Design review of the part built by this model. Coordinates are the model's own, in mm. Face numbers are marked on the shaded views. A direction names the side the tool comes from. Give positions to 0.01 mm unless a question says otherwise; leave off trailing zeros. Loops run counter-clockwise (first coordinate to the right, second up) from the corner with the lowest first, then second, coordinate; pieces in that order, holes last. Notation, with made-up numbers: (50.5, 63.25) - (62.5, 63.25) arc R13 ccw to (62.5, 81.25) - close; hole circle Ø11 at (-13, 41.25). An arc over 180 degrees is marked (long way). Write each question's results on one line, items separated by ' | '.
from build123d import *

# Parameters (mm, degrees)
F2_R     = 4
F3_R     = 1
F4_R     = 2
F5_DEPTH = 25


with BuildPart() as f1:
    # F0 (on Top) → F1 (revolve)
    with BuildSketch(Plane.XY):
        with BuildLine():
            Line((37.5, -2.6), (37.5, 0))
            Line((37.5, 0), (46.8, 0))
            Line((46.8, 0), (46.8, 0.65))
            Line((46.8, 0.65), (38.4, 0.65))
            Line((38.4, 0.65), (38.4, 2.3))
            Line((38.4, 2.3), (34.8, 2.3))
            Line((34.8, 2.3), (34.8, 7))
            Line((34.8, 7), (21.576792, 14.108865))
            Line((21.576792, 14.108865), (18.7, 17))
            Line((18.7, 17), (18.7, 33))
            Line((18.7, 33), (0, 33))
            Line((0, 33), (0, 7.885643))
            ThreePointArc((0, 7.885643), (5.193057, 8.584234), (10.016886, 10.630338))
            Line((10.016886, 10.630338), (32.484462, 0))
            Line((32.484462, 0), (35.5, 0))
            Line((35.5, 0), (35.5, -2.6))
            Line((35.5, -2.6), (37.5, -2.6))
        make_face()
    revolve(axis=Axis((0, 27.784977, 0), (0, 1, 0)))

    # F2
    f2_edges = [f1.edges().sort_by_distance(p)[0] for p in [
        (-18.7, 33, 0),
    ]]
    fillet(f2_edges, radius=F2_R)

    # F3
    f3_edges = [f1.edges().sort_by_distance(p)[0] for p in [
        (-34.8, 7, 0),
        (-34.8, 2.3, 0),
    ]]
    fillet(f3_edges, radius=F3_R)

    # F4 (on face) → F5 (cut)
    with BuildSketch(Plane.XZ):
        with BuildLine():
            ThreePointArc((0, -46.8), (33.092597, -33.092597), (46.8, 0))
            ThreePointArc((46.8, 0), (46.300332, -3.839319), (44.834617, -7.422853))
            ThreePointArc((44.834617, -7.422853), (28.647845, -28.647845), (7.422853, -44.834618))
            ThreePointArc((7.422853, -44.834618), (3.839319, -46.300332), (0, -46.8))
        make_face()
        with BuildLine():
            ThreePointArc((-44.834618, -7.422853), (-46.300332, -3.839319), (-46.8, 0))
            ThreePointArc((-46.8, 0), (-33.092597, -33.092597), (0, -46.8))
            ThreePointArc((0, -46.8), (-3.839319, -46.300332), (-7.422853, -44.834618))
            ThreePointArc((-7.422853, -44.834618), (-28.647845, -28.647845), (-44.834618, -7.422853))
        make_face()
        with BuildLine():
            ThreePointArc((-7.422852, 44.834618), (-3.839319, 46.300332), (0, 46.8))
            ThreePointArc((0, 46.8), (-33.092597, 33.092597), (-46.8, 0))
            ThreePointArc((-46.8, 0), (-46.300332, 3.839319), (-44.834618, 7.422853))
            ThreePointArc((-44.834618, 7.422853), (-28.647845, 28.647845), (-7.422852, 44.834618))
        make_face()
        with BuildLine():
            ThreePointArc((0, 46.8), (3.839319, 46.300332), (7.422853, 44.834618))
            ThreePointArc((7.422853, 44.834618), (28.647845, 28.647845), (44.834618, 7.422853))
            ThreePointArc((44.834618, 7.422853), (46.300332, 3.839319), (46.8, 0))
            ThreePointArc((46.8, 0), (33.092597, 33.092597), (0, 46.8))
        make_face()
        with Locations((0, -42)):
            Circle(F4_R)
        with Locations((0, 42)):
            Circle(F4_R)
        with Locations((-42, 0)):
            Circle(F4_R)
        with Locations((42, 0)):
            Circle(F4_R)
    extrude(amount=-F5_DEPTH, mode=Mode.SUBTRACT)


solid = f1.part
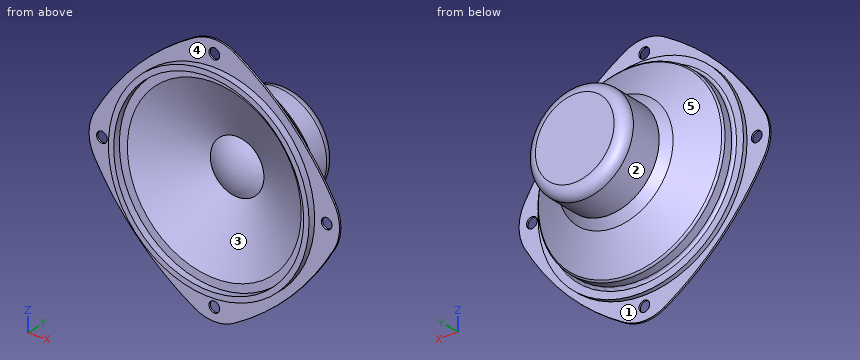
(1) Take a section at A-A on x = -42. Give the boundary of the cut face in (y, z).
Answers below:
outline: (0, -12.1) - (0.65, -12.1) - (0.65, -2) - (0, -2) - close; (0, 2) - (0.65, 2) - (0.65, 12.1) - (0, 12.1) - close
(2) Wall thickness on line 1 along Z through (x, y) = (0, -1.6); line 2 along Z through (x, y) = (-3, 1); line 3 along Z through (x, y) = (15, 29.5): over which ranges is each line inside the solid? List them lowest first. Write a range as from..to.
Answers below:
line 1: -37.5..-35.5, 35.5..37.5 | line 2: -38.28..-30.22, 30.22..38.28 | line 3: -11.11..11.11
(3) Insertion check: P1, Ø6.5, axis at x = 0, z = -42, coming from the +Y side; P2, Ø12, axis at y = 1, z = -36.5, coming from the +X side; P3, Ø12, axis at x = -14.5, y = 24, coming from the +Z side; P4, Ø3, axis at x = 42, z = 0, coming from the +Y side. Each pin has a flat end and moves straight along its axis. Give the tip position at first contact, or say it passes through.
Answers below:
P1: y = 0.65 | P2: x = 26.74 | P3: z = 16.66 | P4: through
(4) Take a section at C-C on y = 5. Give the boundary of the cut face in (x, z).
Answers below:
outline: circle Ø69.6 at (0, 0); hole circle Ø43.83 at (0, 0)
(5) Take a section at B-B on z = 42. Give the boundary of the cut face in (x, y), plus the area to 3 significant figures.
Answers below:
outline: (-12.1, 0) - (-2, 0) - (-2, 0.65) - (-12.1, 0.65) - close; (2, 0) - (12.1, 0) - (12.1, 0.65) - (2, 0.65) - close | area: 13.1 mm2
(6) Draft analysis for pull direction Z (two halves, no side actions). For the marked faces 1, 2 and 3, state which applies: pulls with the +Z half, pulls with the -Z half, needs draft (parallel to the pull), parting line crosses it, or undercut.
Answers below:
face 1: needs draft | face 2: parting line crosses it | face 3: undercut
(7) Tool access review of the marked faces 4 and 5: name each direction out of +Z, -Z, +X, -X, +Y, -Y from which nothing blocks a thin tool from reaching the whole face with its end or side.
Answers below:
face 4: -Y | face 5: +Y
